Drawing for the job (mm, zero at the part's lowest x, y, z). A direction names the side the tool comes from. Coordinates: 2 decimals unless noted, no trailing zeros. Write each loop counter-clockwise with the first axis right and the second up, starting at its lowest first coordinate (ties: lowest second). Pieces come first, ordered by that corner, then holes. Notation, with made-up numbers: M -27.5,82 L -11.5,82 A16 cw -11.5,106 Z; hole C 89.5,40.25 d1. An arc over 180 degrees is marked long. Put each result on its own line as item: value. Start each with the question number.
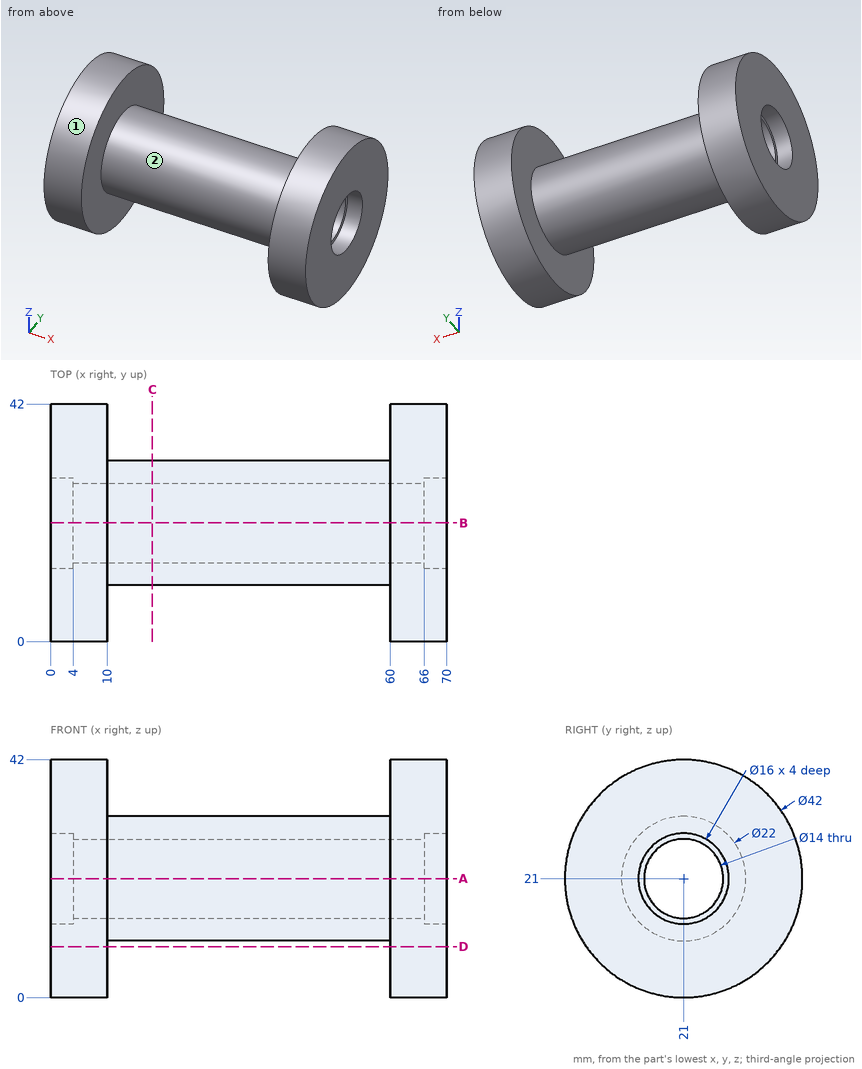
(1) Slice it at C-C, the plane x = 18. Write the cut outline in (y, z), then the cut area to 3 significant figures.
(2) Slice it at A-A, the plane z = 21. Write the cut outline in (x, y), then the cut area to 3 significant figures.
(3) Which spindle directions (+Z, -Z, +X, -X, +Y, -Y) get a long thin tool onto all of the face, cutting with end or side? Do the marked faces 1 and 2. Say none if no direction does.
(4) Drill centre lines: line 1 (X direction, y = 34, z = 33); line 2 (Z direction, x = 34.5, y = 21); line 3 (Y direction, x = 62, z = 21). Where is each one in solid material? Low to high. Write a range as [from, to].
(5) Slice it at D-D, the plane z = 9. Write the cut outline in (x, y), then the cut area to 3 significant figures.
(6) Drop flat-ended pins along their axis: pin 1 (14.5 mm diameter, centred on y = 21, z = 21, fed in from -X); pin 2 (2 mm diameter, centred on x = 25, y = 10, fed in from +Z); pin 3 (1 mm diameter, centred on x = 10, y = 10, fed in from -Z). Give the stop position or say it passes through.
Result set:
1. outline: C 21,21 d22; hole C 21,21 d14
1. area: 226 mm^2
2. outline: M 0,0 L 10,0 L 10,10 L 60,10 L 60,0 L 70,0 L 70,13 L 66,13 L 66,14 L 4,14 L 4,13 L 0,13 Z; M 0,29 L 4,29 L 4,28 L 66,28 L 66,29 L 70,29 L 70,42 L 60,42 L 60,32 L 10,32 L 10,42 L 0,42 Z
2. area: 944 mm^2
3. face 1: +X, -X
3. face 2: none
4. line 1: x = [0, 10], [60, 70]
4. line 2: z = [10, 14], [28, 32]
4. line 3: y = [0, 14], [28, 42]
5. outline: M 0,3.77 L 10,3.77 L 10,38.23 L 0,38.23 Z; M 60,3.77 L 70,3.77 L 70,38.23 L 60,38.23 Z
5. area: 689 mm^2
6. pin 1: stops at x = 4
6. pin 2: stops at z = 25.58
6. pin 3: stops at z = 2.81
